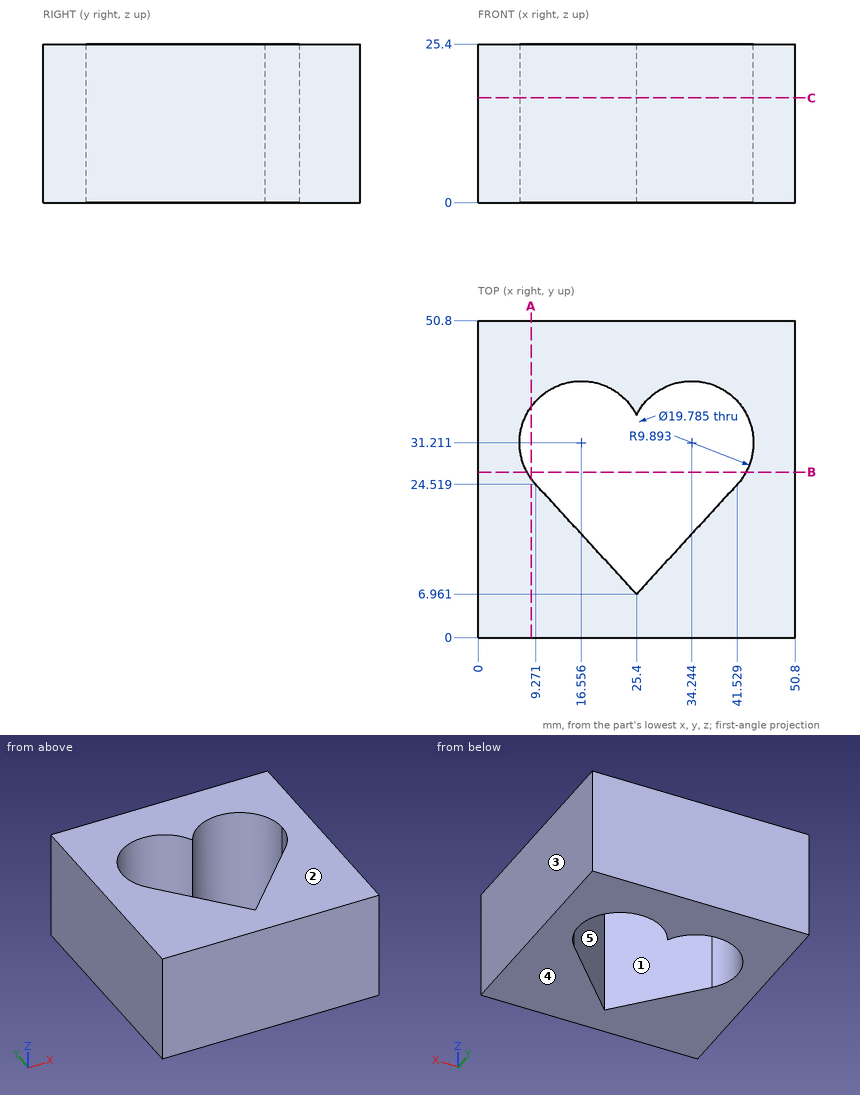
Drawing for the job (mm, zero at the part's lowest x, y, z). A direction names the side the tool comes from. Coordinates: 2 decimals unless noted, no trailing zeros. Write each loop counter-clockwise with the first axis right and the second up, starting at its lowest first coordinate (ties: lowest second). Pieces come first, ordered by that corner, then holes. Notation, with made-up numbers: (66.5, -36.75) - (121.5, -36.75) arc R14 cw to (121.5, -22.75) - close; hole circle Ø10 at (-24.75, 65). An arc over 180 degrees is marked (long way). Write each question's results on one line, items separated by ' | '. Start each with the question number.
1) Probe line 1 along X through (y, z) = (38, 19); line 2 along X through (y, z) = (38.5, 5) (1 decimal); line 3 along Y through (x, z) = (39.5, 18). List the from-to ranges inside material, lowest first. Write a range as from..to.
2) 3-axis set-ups, long thin cutter, end or side, ignore diameter. For the marked faces 4 and 5: which of +Z, -Z, +X, -X, +Y, -Y reach the whole face in a straight line?
3) Cut at A-A (x = 8.5). Write the cut outline in (y, z), then the cut area to 3 significant figures.
4) Cut at C-C (z = 16.75). Write the cut outline in (x, y) (1 decimal), then the cut area to 3 significant figures.
5) Mould opens along X. For the marked faces 1, 2 and 3 say: pulls with the +X half, pulls with the -X half, needs draft (parallel to the pull), parting line crosses it, or undercut.
6) Cut at B-B (y = 26.5). Write the cut outline in (x, z).
Returned:
1) line 1: 0..9.36, 23.75..27.05, 41.44..50.8 | line 2: 0..9.9, 23.2..27.6, 40.9..50.8 | line 3: 0..22.31, 39.59..50.8
2) face 4: -Z, +X, -X, +Y, -Y | face 5: +Z, -Z
3) outline: (0, 0) - (25.47, 0) - (25.47, 25.4) - (0, 25.4) - close; (36.95, 0) - (50.8, 0) - (50.8, 25.4) - (36.95, 25.4) - close | area: 999 mm^2
4) outline: (0, 0) - (50.8, 0) - (50.8, 50.8) - (0, 50.8) - close; hole (9.3, 24.5) - (25.4, 7) - (41.5, 24.5) arc R9.9 ccw to (44.1, 31.2) arc R9.9 ccw to (25.4, 35.6) arc R9.9 ccw (long way) to start | area: 1,760 mm^2
5) face 1: undercut | face 2: needs draft | face 3: pulls with the +X half
6) outline: (0, 0) - (7.86, 0) - (7.86, 25.4) - (0, 25.4) - close; (42.94, 0) - (50.8, 0) - (50.8, 25.4) - (42.94, 25.4) - close
